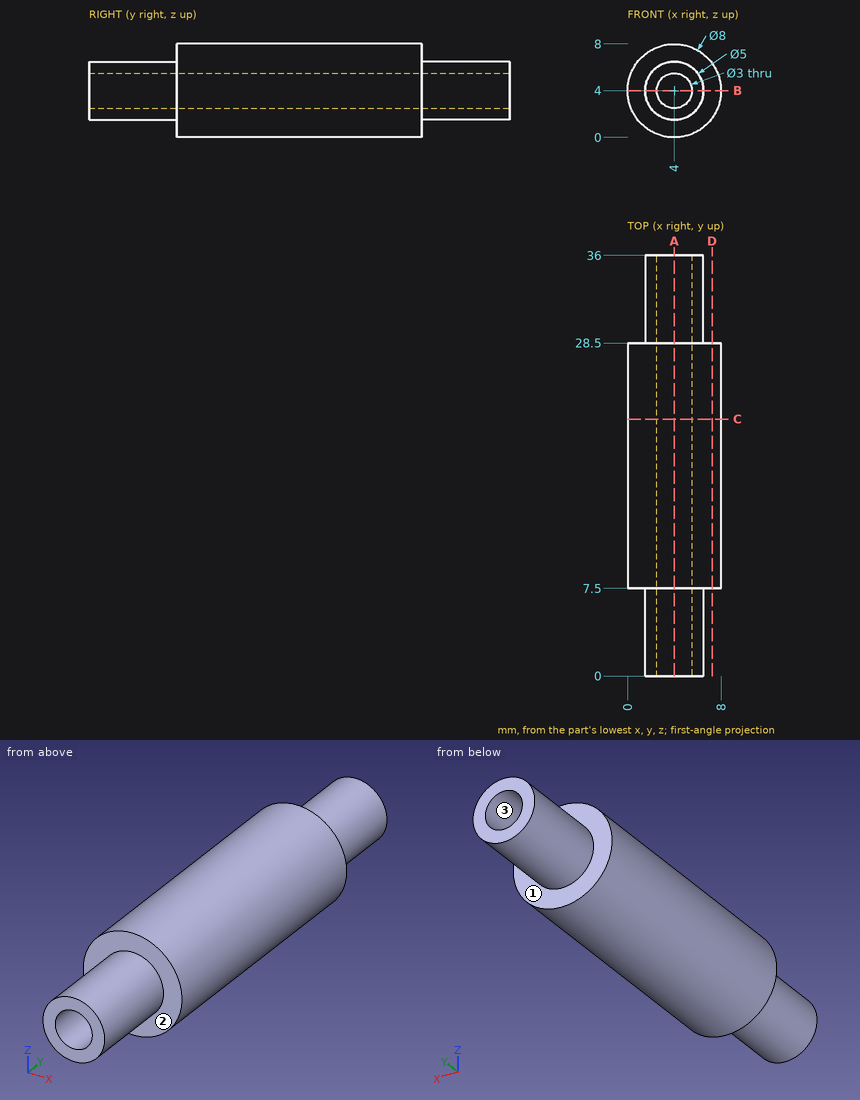
For this review, use the dimensioned drawing (mm, ordinates from the lowest corner) and the shaded views. A direction names the side the tool comes from. Give positions to 0.01 mm unless a question says otherwise; leave off trailing zeros. Write each loop counter-clockwise with the first axis right and the second up, starting at its lowest first coordinate (ties: lowest second). Pieces come first, ordered by that corner, then holes. Notation, with made-up numbers: M 32,50.25 L 82,50.25 A11 cw 82,60.25 Z; hole C -26,72 d9. An arc over 180 degrees is marked long. Answer as a JSON object with one key per item and string values. Group by question number.
1) We need section D-D (x = 7.25). Give the boundary of the cut face in (y, z), and give its area (3 significant figures).
2) We need section A-A (x = 4). Give the boundary of the cut face in (y, z).
3) We need section B-B (z = 4). Give the boundary of the cut face in (x, y), and give its area (3 significant figures).
4) Tool access review of the marked faces 1, 2 and 3: name each direction out of +Z, -Z, +X, -X, +Y, -Y from which nothing blocks a thin tool from reaching the whole face with its end or side.
5) We need section C-C (y = 22). Give the boundary of the cut face in (x, z).
6) For line 1 along X through (y, z) = (26, 4); line 2 along X through (y, z) = (29.5, 4), list the stretches that pass through material, from the lowest coordinate up.
Answer key:
{
 "1": {"outline": "M 7.5,1.67 L 28.5,1.67 L 28.5,6.33 L 7.5,6.33 Z", "area": "97.9 mm²"},
 "2": {"outline": "M 0,1.5 L 7.5,1.5 L 7.5,0 L 28.5,0 L 28.5,1.5 L 36,1.5 L 36,2.5 L 0,2.5 Z; M 0,5.5 L 36,5.5 L 36,6.5 L 28.5,6.5 L 28.5,8 L 7.5,8 L 7.5,6.5 L 0,6.5 Z"},
 "3": {"outline": "M 0,7.5 L 1.5,7.5 L 1.5,0 L 2.5,0 L 2.5,36 L 1.5,36 L 1.5,28.5 L 0,28.5 Z; M 5.5,0 L 6.5,0 L 6.5,7.5 L 8,7.5 L 8,28.5 L 6.5,28.5 L 6.5,36 L 5.5,36 Z", "area": "135 mm²"},
 "4": {"face 1": "+Y", "face 2": "-Y", "face 3": "+Y, -Y"},
 "5": {"outline": "C 4,4 d8; hole C 4,4 d3"},
 "6": {"line 1": "x = 0 to 2.5, 5.5 to 8", "line 2": "x = 1.5 to 2.5, 5.5 to 6.5"}
}
